Design review of the part built by this model. Coordinates are the model's own, in mm. Face numbers are marked on the shaded views. Coordinates: 2 decimals unless noted, no trailing zeros. Write each loop counter-clockwise with the first axis right and the second up, starting at its lowest first coordinate (ties: lowest second). Pieces come first, ordered by that corner, then holes. Notation, with made-up numbers: M 55.5,9.5 L 61.5,9.5 A19 ccw 61.5,17.5 Z; hole C 28.25,20 d2. An arc over 180 degrees is marked long. Write item = value, one per line.
```python
from build123d import *

# Parameters (mm, degrees)
SKETCH1_W           = 67
SKETCH1_H           = 74.4
BOSS_EXTRUDE1_DEPTH = 22
FILLET1_R           = 10
SKETCH2_W           = 15
SKETCH2_H           = 13
SKETCH2_W_2         = 10
SKETCH2_H_2         = 5
CUT_EXTRUDE1_DEPTH  = 10
SKETCH3_W           = 2
SKETCH3_H           = 14
SKETCH3_H_2         = 24
BOSS_EXTRUDE2_DEPTH = 1


with BuildPart() as part:
    # Sketch1 → Boss-Extrude1 (new body)
    with BuildSketch(Plane(origin=(0, 0, 0), x_dir=(1, 0, 0), z_dir=(0, 1, 0))):
        Rectangle(SKETCH1_W, SKETCH1_H)
    extrude(amount=BOSS_EXTRUDE1_DEPTH)

    # Fillet1
    fillet1_edges = [part.edges().sort_by_distance(p)[0] for p in [
        (33.5, 11, 37.2),
        (-33.5, 11, 37.2),
        (-33.5, 11, -37.2),
        (33.5, 11, -37.2),
    ]]
    fillet(fillet1_edges, radius=FILLET1_R)

    # Sketch2 → Cut-Extrude1 (cut)
    with BuildSketch(Plane(origin=(0, 0, -37.2), x_dir=(-1, 0, 0), z_dir=(0, 0, -1))):
        with Locations((-5, 12.5)):
            Rectangle(SKETCH2_W, SKETCH2_H)
        with Locations((10.5, 7.5)):
            Rectangle(SKETCH2_W_2, SKETCH2_H_2)
    extrude(amount=-CUT_EXTRUDE1_DEPTH, mode=Mode.SUBTRACT)

    # Sketch3 → Boss-Extrude2 (add)
    with BuildSketch(Plane(origin=(0, 22, 0), x_dir=(1, 0, 0), z_dir=(0, 1, 0))):
        with Locations((25, 18.2)):
            Rectangle(SKETCH3_W, SKETCH3_H)
        with Locations((25, -2.8)):
            Rectangle(SKETCH3_W, SKETCH3_H_2)
    extrude(amount=BOSS_EXTRUDE2_DEPTH)


solid = part.part
```
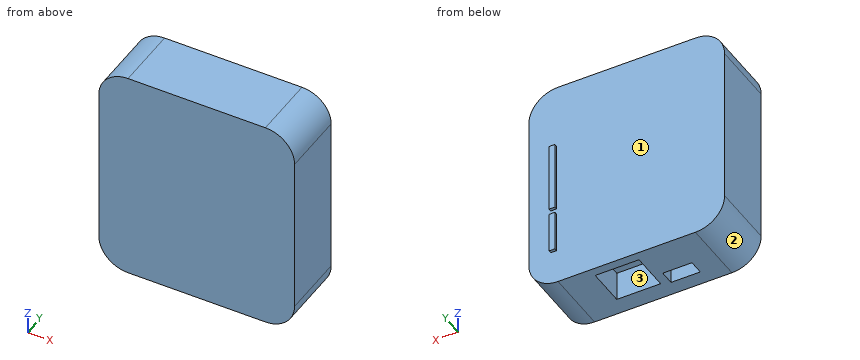
Q1. The part is to be moulded in two halves that separate along X. For the marked faces 1, 2 and 3, say which applies: +X half, -X half, draft (parallel to the pull), parting line (faces both ways), or undercut.
Check result:
face_1 = draft
face_2 = -X half
face_3 = undercut
Q2. Wall thickness on line 1 (Y direction, x = 21.5, z = -20); line 2 (Z direction, x = 11.5, y = 18); line 3 (X direction, y = 15.5, z = -34): over which ranges is each line inside the solid? List them lowest first.
Check result:
line_1 = 0 to 22
line_2 = -27.2 to 37.2
line_3 = -30.83 to -2.5, 12.5 to 30.83
Q3. Consider section C-C, the plane x = 2. State the section outline as (y, z) points.
Check result:
outline = M 0,-37.2 L 6,-37.2 L 6,-27.2 L 19,-27.2 L 19,-37.2 L 22,-37.2 L 22,37.2 L 0,37.2 Z
Q4. For P1, Ø10.5, axis at x = 6.5, y = 13, coming from the -Z side; P2, Ø0.8, axis at y = 22.5, z = -21, coming from the +X side; P3, Ø0.5, axis at x = 24.5, y = 22.5, coming from the +Z side, all flat-tipped, find the tip position at first contact; note any pin that passes through.
Check result:
P1 = -27.2
P2 = 26
P3 = 14.8
Q5. Consider section D-D, the plane x = 13.5. State the section outline as (y, z) points.
Check result:
outline = M 0,-37.2 L 22,-37.2 L 22,37.2 L 0,37.2 Z
Q6. Consider section A-A, the plane z = -7. State the section outline as (x, y) points.
Check result:
outline = M -33.5,0 L 33.5,0 L 33.5,22 L 26,22 L 26,23 L 24,23 L 24,22 L -33.5,22 Z
Q7. Consider section B-B, the plane y = 11. State the section outline as (x, z) points, and give its area (3 significant figures).
Check result:
outline = M -33.5,-27.2 A10 ccw -23.5,-37.2 L -2.5,-37.2 L -2.5,-27.2 L 12.5,-27.2 L 12.5,-37.2 L 23.5,-37.2 A10 ccw 33.5,-27.2 L 33.5,27.2 A10 ccw 23.5,37.2 L -23.5,37.2 A10 ccw -33.5,27.2 Z
area = 4,750 mm²
